Geometry: see drawing. Coordinates: mm, zero at the bounding-box minimum. Coordinates: 2 decimals unless noted, no trailing zeros. Order: outer loops, then holes, each group sorted by start corner. A loop starts at its lowest first (then second) coordinate and runs counter-clockwise, first axis right, second up.
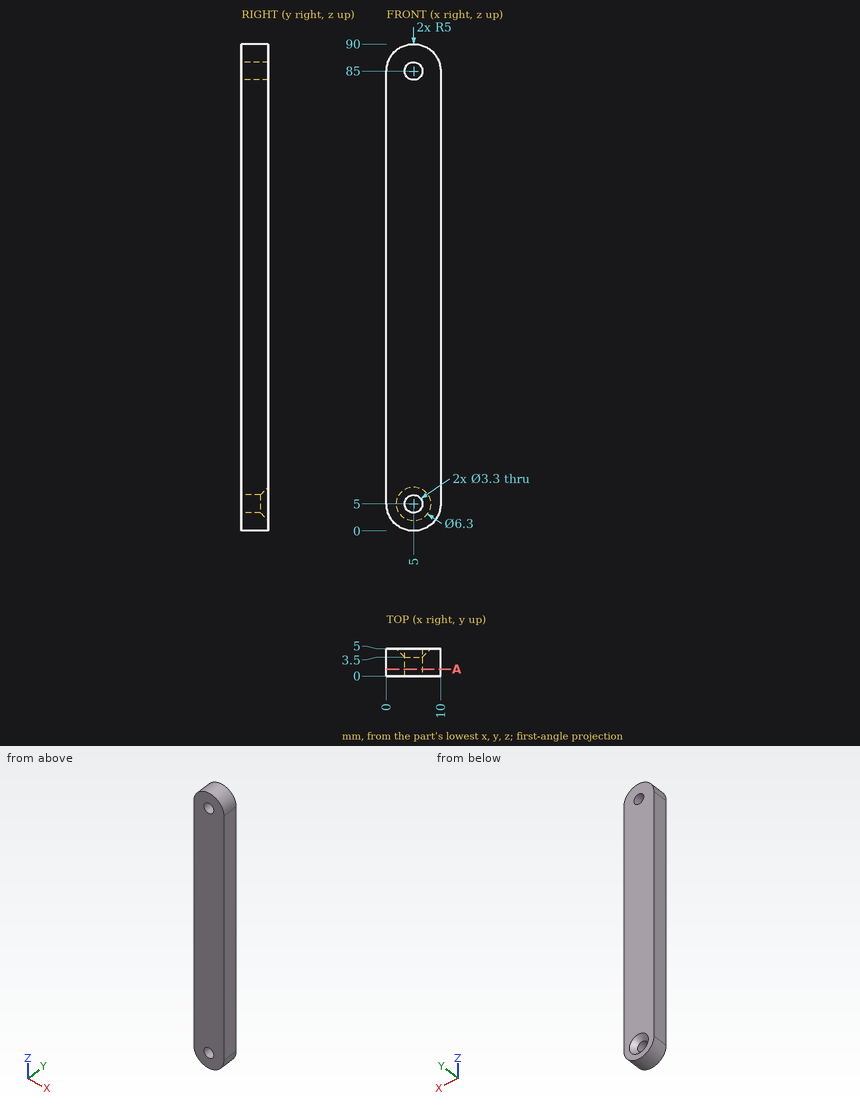
Item 1: Ray query, probe 1 along Z at (x, y) = (5, 1.45); probe 2 along X at (y, z) = (3.65, 85); probe 3 along Z at (x, y) = (4.25, 0.85). Return the intervals inside material, ascending.
Response values:
probe 1: z = 0 to 3.35, 6.65 to 83.35, 86.65 to 90
probe 2: x = 0 to 3.35, 6.65 to 10
probe 3: z = 0.06 to 3.53, 6.47 to 83.53, 86.47 to 89.94
Item 2: Cut plane A-A on y = 1.25. Return loops of the section in (x, z), then the cut area to 3 significant figures.
Response values:
outline: (0, 5) arc R5 ccw to (10, 5) - (10, 85) arc R5 ccw to (0, 85) - close; hole circle Ø3.3 at (5, 5); hole circle Ø3.3 at (5, 85)
area: 861 mm2
Item 3: Pin query (flat end, axial travel): pin 1 Ø3 at (y, z) = (2, 20.5) entering from -X; pin 2 Ø3 at (x, y) = (1, 4.5) entering from -Z. Return the tip coordinate at first contact, or that it passes through.
Response values:
pin 1: stops at x = 0
pin 2: stops at z = 0.67
